from build123d import *

# Parameters (mm, degrees)
SKETCH2_W                = 13.081
SKETCH2_H                = 31.623
BOSS_EXTRUDE1_DEPTH      = 1.524
BOSS_EXTRUDE3_DEPTH      = 0.508
BOSS_EXTRUDE3_DEPTH_BACK = 4.064
SKETCH3_R                = 0.375
CHAMFER2_SIZE            = 0.127
SKETCH4_W                = 1.27
SKETCH4_H                = 2.54
BOSS_EXTRUDE4_DEPTH      = 0.762
SKETCH5_W                = 5.08
SKETCH5_H                = 3.81
BOSS_EXTRUDE5_DEPTH      = 1.524
SKETCH6_R                = 1.462847535
SKETCH6_R_2              = 1.470158192
CUT_EXTRUDE1_DEPTH       = 1.524


with BuildPart() as part:
    # Sketch2 → Boss-Extrude1 (new body)
    with BuildSketch(Plane(origin=(0, 0, 0), x_dir=(1, 0, 0), z_dir=(0, 1, 0))):
        with Locations((6.5405, 15.8115)):
            Rectangle(SKETCH2_W, SKETCH2_H)
    extrude(amount=BOSS_EXTRUDE1_DEPTH)

    # Sketch3 → Boss-Extrude3 (add, two sides: drawn at the far end of the back side and taken through both)
    with BuildSketch(Plane(origin=(0, 1.524, 0), x_dir=(1, 0, 0), z_dir=(0, 1, 0)).offset(-BOSS_EXTRUDE3_DEPTH_BACK)):
        with Locations(Location((3.81, 28.623, 0), (0, 0, 90))):
            Circle(SKETCH3_R)
        with Locations(Location((6.35, 28.623, 0), (0, 0, 90))):
            Circle(SKETCH3_R)
        with Locations(Location((8.89, 28.623, 0), (0, 0, 90))):
            Circle(SKETCH3_R)
        with Locations(Location((3.81, 4.445, 0), (0, 0, 90))):
            Circle(SKETCH3_R)
        with Locations(Location((9.01, 4.445, 0), (0, 0, 90))):
            Circle(SKETCH3_R)
    extrude(amount=BOSS_EXTRUDE3_DEPTH + BOSS_EXTRUDE3_DEPTH_BACK)

    # Chamfer2
    chamfer2_edges = [part.edges().sort_by_distance(p)[0] for p in [
        (3.81, 1.524, -28.248),
        (3.81, 0, -28.248),
        (3.81, -2.54, -28.248),
        (3.81, 2.032, -28.248),
        (6.35, 1.524, -28.248),
        (6.35, 0, -28.248),
        (6.35, -2.54, -28.248),
        (6.35, 2.032, -28.248),
        (8.89, 1.524, -28.248),
        (8.89, 0, -28.248),
        (8.89, -2.54, -28.248),
        (8.89, 2.032, -28.248),
        (3.81, 1.524, -4.07),
        (3.81, -2.54, -4.07),
        (3.81, 2.032, -4.07),
        (9.01, 1.524, -4.07),
        (9.01, -2.54, -4.07),
        (9.01, 2.032, -4.07),
    ]]
    chamfer(chamfer2_edges, length=CHAMFER2_SIZE)

    # Sketch4 → Boss-Extrude4 (add)
    with BuildSketch(Plane(origin=(0, 1.524, 0), x_dir=(1, 0, 0), z_dir=(0, 1, 0))):
        with Locations((1.778, 21.463)):
            Rectangle(SKETCH4_W, SKETCH4_H)
        with Locations((5.08, 21.463)):
            Rectangle(SKETCH4_W, SKETCH4_H)
        with Locations((8.382, 21.463)):
            Rectangle(SKETCH4_W, SKETCH4_H)
        with Locations((11.684, 21.463)):
            Rectangle(SKETCH4_W, SKETCH4_H)
    extrude(amount=BOSS_EXTRUDE4_DEPTH)

    # Sketch5 → Boss-Extrude5 (add)
    with BuildSketch(Plane(origin=(0, 1.524, 0), x_dir=(1, 0, 0), z_dir=(0, 1, 0))):
        with Locations((6.35, 14.224)):
            Rectangle(SKETCH5_W, SKETCH5_H)
    extrude(amount=BOSS_EXTRUDE5_DEPTH)

    # Sketch6 → Cut-Extrude1 (cut)
    with BuildSketch(Plane(origin=(0, 1.524, 0), x_dir=(1, 0, 0), z_dir=(0, 1, 0))):
        with Locations(Location((2.030479475, 14.174875331, 0), (0, 0, 270))):
            Circle(SKETCH6_R)
        with Locations(Location((11.138543977, 14.174875331, 0), (0, 0, 270))):
            Circle(SKETCH6_R_2)
    extrude(amount=-CUT_EXTRUDE1_DEPTH, mode=Mode.SUBTRACT)


solid = part.part
Can you work these out from the model? Positions are in its coordinate system, mm. A direction names the side the tool comes from. Give positions to 0.01 mm unless a question says otherwise; leave off trailing zeros. Loops run counter-clockwise (first coordinate to the right, second up) from the corner with the lowest first, then second, coordinate; pieces in that order, holes last. Notation, with made-up numbers: (67, 54.5) - (100, 54.5) arc R16 ccw to (100, 67.5) - close; hole circle Ø11 at (0.25, 65). An arc over 180 degrees is marked (long way). Return JSON: item names as keys, results as strings.
1. I want a section at B-B on y = -1.9. Please give me the cut outline in (x, z) (3 decimals), and give its area (3 significant figures).
Output values:
{"outline": "circle Ø0.75 at (3.81, -28.623); circle Ø0.75 at (3.81, -4.445); circle Ø0.75 at (6.35, -28.623); circle Ø0.75 at (8.89, -28.623); circle Ø0.75 at (9.01, -4.445)", "area": "2.21 mm²"}
2. I want a section at C-C on z = -22. Please give me the cut outline in (x, y) (3 decimals).
Output values:
{"outline": "(0, 0) - (13.081, 0) - (13.081, 1.524) - (12.319, 1.524) - (12.319, 2.286) - (11.049, 2.286) - (11.049, 1.524) - (9.017, 1.524) - (9.017, 2.286) - (7.747, 2.286) - (7.747, 1.524) - (5.715, 1.524) - (5.715, 2.286) - (4.445, 2.286) - (4.445, 1.524) - (2.413, 1.524) - (2.413, 2.286) - (1.143, 2.286) - (1.143, 1.524) - (0, 1.524) - close"}
3. For faces 5 (the face through (8.89, 2, -14)), 6 (the face through (3.81, 2, -14)), 7 (the face through (6, 1, -31.623)), which set-ups out of +Z, -Z, +X, -X, +Y, -Y let a thin tool reach every point of the face, with its end or its side?
Output values:
{"face 5": "+X, +Y", "face 6": "-X, +Y", "face 7": "-Z, +X, -X, +Y, -Y"}
4. I'm going to push flat-ended pins straight in: pin 1 Ø5 at (x, z) = (10, -22.5) entering from +Y; pin 2 Ø2 at (x, z) = (11.5, -17) entering from +Y; pin 3 Ø0.8 at (y, z) = (2, -22) entering from +X; pin 4 Ø4 at (x, z) = (2.03, -14.17) entering from +Y. Where does each tip first touch, or does it pass through?
Output values:
{"pin 1": "stops at y = 2.29", "pin 2": "stops at y = 1.52", "pin 3": "stops at x = 12.32", "pin 4": "stops at y = 3.05"}
5. If I drill on line 1 (Y direction, x = 2.5, z = -4); line 2 (Y direction, x = 6.5, z = -15); line 3 (Z direction, x = 1.75, y = 0.55), over which ranges is the centre line in solid material (lowest first)?
Output values:
{"line 1": "y = 0 to 1.52", "line 2": "y = 0 to 3.05", "line 3": "z = -31.62 to -15.61, -12.74 to 0"}
6. We'd pull the mould along Z, two halves only. Please class faces 1 (the face through (6, 1, 0)), 2 (the face through (11.203, 0.773, -15.644)), 3 (the face through (6, 2, -16.129)), 4 (the face through (8, 2.286, -21)): +Z half, -Z half, draft (parallel to the pull), parting line (faces both ways), or undercut.
Output values:
{"face 1": "+Z half", "face 2": "undercut", "face 3": "undercut", "face 4": "draft"}
7. I want a section at A-A on x = 10.5. Please give me the cut outline in (y, z), and give its area (3 significant figures).
Output values:
{"outline": "(0, -31.62) - (1.52, -31.62) - (1.52, -15.5) - (0, -15.5) - close; (0, -12.85) - (1.52, -12.85) - (1.52, 0) - (0, 0) - close", "area": "44.2 mm²"}
8. I want a section at D-D on y = 1.05. Please give me the cut outline in (x, z).
Output values:
{"outline": "(0, -31.62) - (13.08, -31.62) - (13.08, 0) - (0, 0) - close; hole circle Ø2.93 at (2.03, -14.17); hole circle Ø2.94 at (11.14, -14.17)"}
